from build123d import *

# Parameters (mm, degrees)
F0_W     = 260.35
F0_H     = 203.2
F1_DEPTH = 203.2
F2_R     = 31.75
F4_DEPTH = 203.201


with BuildPart() as f1:
    # F0 (on Top) → F1 (new body)
    with BuildSketch(Plane.XY):
        with Locations((-43.21573, 7.619998)):
            Rectangle(F0_W, F0_H)
    extrude(amount=F1_DEPTH)

    # F2
    f2_edges = [f1.edges().sort_by_distance(p)[0] for p in [
        (-173.39073, 109.219998, 101.6),
        (-173.39073, -93.980002, 101.6),
        (86.95927, 109.219998, 101.6),
        (86.95927, -93.980002, 101.6),
    ]]
    fillet(f2_edges, radius=F2_R)

    # F3 (on face) → F4 (cut, through all)
    with BuildSketch(Plane.XZ.offset(93.980002)):
        Polygon((19.64927, 203.2), (-106.08073, 203.2), (-86.431459, 187.104467), (0, 187.104467), align=None)
        Polygon((-101.357388, 10.098124), (-117.510729, 0), (31.106714, 0), (14.953374, 10.098124), align=None)
    extrude(amount=-F4_DEPTH, mode=Mode.SUBTRACT)

    # F7: sweep along a path in F5
    with BuildLine(Plane.XY.offset(203.2)) as f7_path:
        ThreePointArc((20.038901, -93.980002), (29.431866, 7.632308), (19.77627, 109.219998))
        Line((19.77627, 109.219998), (14.249222, 138.23534))
    # F6 (on face) → F7 (sweep, cut)
    with BuildSketch(Plane.XZ.offset(93.980002)):
        Polygon((0, 187.104467), (19.64927, 203.2), (0, 203.2), (-25.094712, 203.330889), (-25.094712, 187.104467), align=None)
    sweep(path=f7_path.line, mode=Mode.SUBTRACT)


solid = f1.part
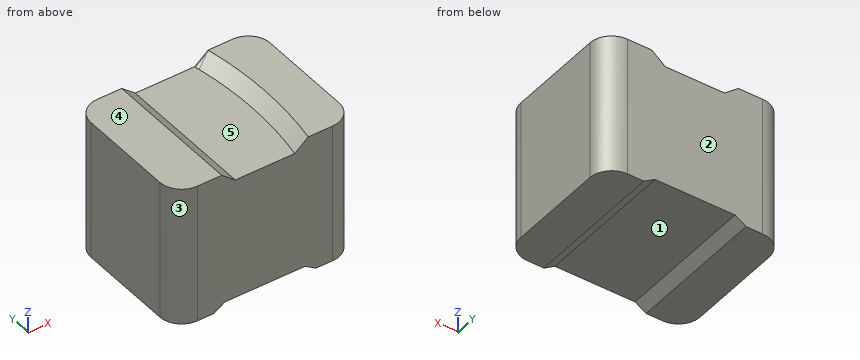
Geometry: final body of the model. Coordinates: model frame, mm. Face numbers are marked on the shaded views. A direction names the side the tool comes from. Coordinates: 2 decimals unless noted, no trailing zeros. Order: outer loops, then holes, each group sorted by start corner. A loop starts at its lowest first (then second) coordinate and runs counter-clockwise, first axis right, second up.
1) Section B-B (x = -75). Return loops of the section in (y, z), then the cut area to 3 significant figures.
Result sheet:
outline: (-93.98, 10.1) - (109.22, 10.1) - (109.22, 187.1) - (-93.98, 187.1) - close
area: 36,000 mm2
2) Set-up query: the marked faces 1 and 2. Return all of +Z, -Z, +X, -X, +Y, -Y with unobstructed straight access to the full face (end or side cutting, diameter ignored); none if empty.
Result sheet:
face 1: -Z, +Y, -Y
face 2: +Z, -Z, +X, -X, +Y
3) Section A-A (z = 104). Return loops of the section in (x, y), then the cut area to 3 significant figures.
Result sheet:
outline: (-173.39, -62.23) arc R31.75 ccw to (-141.64, -93.98) - (55.21, -93.98) arc R31.75 ccw to (86.96, -62.23) - (86.96, 77.47) arc R31.75 ccw to (55.21, 109.22) - (-141.64, 109.22) arc R31.75 ccw to (-173.39, 77.47) - close
area: 52,000 mm2
4) Section C-C (x = 65.5). Return loops of the section in (y, z).
Result sheet:
outline: (-92.27, 0) - (107.51, 0) - (107.51, 203.2) - (-92.27, 203.2) - close
5) First-contact query: P1, Ø2, axis at x = 5.5, y = 54.5, coming from the +Z side; P2, Ø3, axis at y = -72.5, z = 120, coming from the -X side; P3, Ø5, axis at x = -60, y = -43.5, coming from the -Z side. Flat tips, straight axial feed; report the tip coordinate or a pass-through.
Result sheet:
P1: stops at z = 187.1
P2: stops at x = -172.16
P3: stops at z = 10.1
6) Draft query along X for the marked faces 3, 4 and 5. Return one class per face: released by +X, released by -X, zero draft, split by the parting line, or undercut.
Result sheet:
face 3: released by -X
face 4: zero draft
face 5: undercut
7) Ray query, probe 1 along Z at (x, y) = (-13, 54); probe 2 along X at (y, z) = (89.5, 79); probe 3 along Z at (x, y) = (30.5, 6.5). Return the intervals inside material, ascending.
Result sheet:
probe 1: z = 10.1 to 187.1
probe 2: x = -171.02 to 84.59
probe 3: z = 0.38 to 203.2
